Autodesk Inventor part; units mm, degrees
ref_plane "YZ Plane" through (0, 0, 0) normal (1, 0, 0) x (0, 1, 0)
ref_plane "XZ Plane" through (0, 0, 0) normal (0, 1, 0) x (-1, 0, 0)
ref_plane "XY Plane" through (0, 0, 0) normal (0, 0, 1) x (1, 0, 0)
sketch "Sketch1" plane through (0, 0, 0) normal (0, 1, 0) x (-1, 0, 0)
  line L0 (0, 0) -> (31.75, 0)
  line L1 (31.75, 0) -> (31.75, -31.75)
  line L2 (31.75, -31.75) -> (0, -31.75)
  line L3 (0, -31.75) -> (0, 0)
  dimension "d0" = 31.75
  dimension "d1" = 31.75
extrude "Extrusion1" add sketch "Sketch1" along normal blind 19.558
sketch "Sketch2" plane through (0, 19.558, 0) normal (0, 1, 0) x (1, 0, 0)
  line L0 (-31.75, 31.75) -> (-31.75, 0) construction
  line L1 (-31.75, 0) -> (0, 31.75) construction
  circle A0 centre (-15.875, 15.875) radius 11.0808
  point P0 (0, 0)
  dimension "d4" = 22.1615
extrude "Extrusion2" add sketch "Sketch2" along normal blind 25.4
sketch "Sketch3" plane through (-15.875, 44.958, -15.875) normal (0, 1, 0) x (1, 0, 0)
  circle A0 centre (0, 0) radius 8.7313
  circle A1 centre (0, 0) radius 11.0808
  point P0 (15.875, -15.875)
  dimension "d19" = 17.4625
extrude "Extrusion3" cut sketch "Sketch3" against normal through all contours A0
sketch "Sketch4" plane through (-31.75, 0, 0) normal (0, 0, 1) x (1, 0, 0)
  circle A0 centre (15.875, 7.796) radius 11
  line L0 (0, 19.558) -> (31.75, 19.558) construction
  line L1 (15.875, 19.558) -> (15.875, 0) construction
  line L2 (31.75, 0) -> (0, 0) construction
  dimension "d10" = 22
  dimension "d20" = 11.762
extrude "Extrusion4" cut sketch "Sketch4" against normal blind 7
sketch "Sketch5" plane through (0, 0, -31.75) normal (0, 0, -1) x (-1, 0, 0)
  circle A0 centre (15.875, 7.796) radius 11
  point P0 (0, 0)
extrude "Extrusion5" cut sketch "Sketch5" against normal blind 7
sketch "Sketch6" plane through (-15.875, 7.796, -7) normal (0, 0, 1) x (-1, 0, 0)
  circle A0 centre (0, 0) radius 6.35
  point P0 (-15.875, 7.796)
  dimension "d15" = 12.7
extrude "Extrusion6" cut sketch "Sketch6" against normal through all
fillet "Fillet1" radius 0.254 4 edges at (-8.1147, 0, -3.5) (-23.6353, 0, -3.5) (-23.6353, 0, -28.25) (-8.1147, 0, -28.25)
properties part number "bearingholder" material "Aluminum 6061"
The listing builds one solid part. Answer for the finished solid, in the listing's coordinates (mm). A direction names the side the tool comes from. Coordinates: 2 decimals unless noted, no trailing zeros. Loops run counter-clockwise (first coordinate to the right, second up) from the corner with the lowest first, then second, coordinate; pieces in that order, holes last. Notation, with made-up numbers: M -17,-39 L 34,-39 A18 ccw 34,-14 Z; hole C 50.5,30.25 d5. An arc over 180 degrees is marked long. Answer in a Markdown table with one row per item.
1) Determine the mould class of faces 1 (the cylindrical face through (-15.52, 18.79, -3.45)), 2 (the flat face through (0, 10, -16)), 3 (the flat face through (-12.1, 18.3, 0)), 4 (the flat face through (-18, 14, -7)) for opening direction X: released by +X, released by -X, zero draft, split by the parting line, or undercut.
Answers below:
| item | result |
|---|---|
| face 1 | undercut |
| face 2 | released by +X |
| face 3 | zero draft |
| face 4 | undercut |
2) Given pin 1 (15 mm diameter, centred on x = -14.5, y = 9.5, fed in from +Z); pin 2 (16.5 mm diameter, centred on x = -15.875, y = 7.796, fed in from -Z); pin 3 (12 mm diameter, centred on y = 31, z = -20.5, fed in from +X); pin 4 (11.5 mm diameter, centred on x = -15.875, y = 7.796, fed in from +Z), each flat-ended and moving along its own axis, determine where each tip first touches the part or whether it passes through.
Answers below:
| item | result |
|---|---|
| pin 1 | z = -7 |
| pin 2 | z = -24.75 |
| pin 3 | x = -4.79 |
| pin 4 | through |
3) Which of the six approach directions +Z, -Z, +X, -X, +Y, -Y give full straight-line access (tool end or side, diameter ignored) to faces 5 (the flat face through (-13, 14, -24.75)), 6 (the flat face through (-5, 19.558, -12)), 7 (the cylindrical face through (-11.2, 3.5, -8.1))?
Answers below:
| item | result |
|---|---|
| face 5 | -Z |
| face 6 | +Y |
| face 7 | +Z, -Z |
4) Find section D-D (y = 15.5). Determine the outline of the cut face in (x, z) (3 decimals).
Answers below:
| item | result |
|---|---|
| outline | M -31.75,-31.75 L -23.727,-31.75 L -23.727,-24.75 L -8.023,-24.75 L -8.023,-31.75 L 0,-31.75 L 0,0 L -8.023,0 L -8.023,-7 L -23.727,-7 L -23.727,0 L -31.75,0 Z; hole C -15.875,-15.875 d17.463 |
5) Find the intervals of material crossed by probe 1 along Z at (x, y) = (-16, 42.5); probe 2 along X at (y, z) = (14.5, -15.5); probe 3 along Y at (x, z) = (-30, -12.5), in increasing order.
Answers below:
| item | result |
|---|---|
| probe 1 | -26.96 to -24.61, -7.14 to -4.79 |
| probe 2 | -31.75 to -24.6, -7.15 to 0 |
| probe 3 | 0 to 19.56 |
6) Find section B-B (x = -16). Determine the outline of the cut face in (y, z), then the cut area to 3 significant figures.
Answers below:
| item | result |
|---|---|
| outline | M 0,-24.75 L 1.45,-24.75 L 1.45,-24.61 L 0,-24.61 Z; M 0,-7.14 L 1.45,-7.14 L 1.45,-7 L 0,-7 Z; M 14.14,-24.75 L 18.8,-24.75 L 18.8,-31.75 L 19.56,-31.75 L 19.56,-26.96 L 44.96,-26.96 L 44.96,-24.61 L 14.14,-24.61 Z; M 14.14,-7.14 L 44.96,-7.14 L 44.96,-4.79 L 19.56,-4.79 L 19.56,0 L 18.8,0 L 18.8,-7 L 14.14,-7 Z |
| area | 132 mm^2 |
7) Find section C-C (z = -23). Determine the outline of the cut face in (x, y) (3 decimals).
Answers below:
| item | result |
|---|---|
| outline | M -31.75,0 L -20.922,0 L -20.922,3.942 A6.35 cw -20.922,11.65 L -20.922,44.958 L -24.361,44.958 L -24.361,19.558 L -31.75,19.558 Z; M -10.828,0 L 0,0 L 0,19.558 L -7.389,19.558 L -7.389,44.958 L -10.828,44.958 L -10.828,11.65 A6.35 cw -10.828,3.942 Z |
